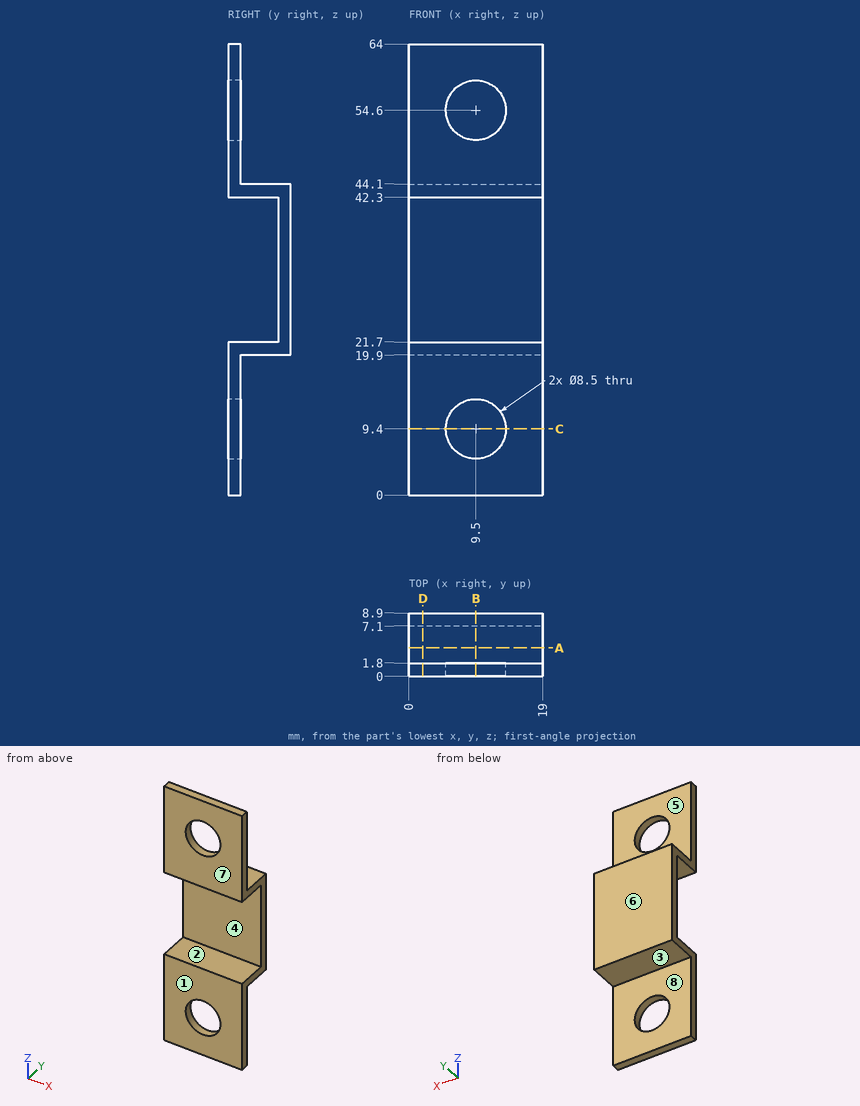
Input: dimensioned drawing with shaded views. Units: mm. Origin: part minimum x, y, z. A direction names the side the tool comes from. Give positions to 0.01 mm unless a question says otherwise; leave off trailing zeros. Loops run counter-clockwise (first coordinate to the right, second up) from the corner with the lowest first, then second, coordinate; pieces in that order, holes last. Notation, with made-up numbers: (-8.5, 42.25) -> (23.5, 42.25) arc R14 ccw to (23.5, 47.25) -> close; hole circle Ø8 at (29, 44.5). An arc over 180 degrees is marked (long way). Use a Markdown table: item, result. Add a question column.
1) Section query D-D, the plane x = 2. Return the cut outline in (y, z).
2) Section query C-C, the plane z = 9.4. Return the cut outline in (x, y), then the cut area to 3 significant figures.
3) Line query: line 1 along Z through (x, y) = (10.5, 1); line 2 along Z through (x, y) = (9.25, 4.5); line 3 along X through (y, z) = (1.45, 9.4). Output: solid intervals per line, ascending. Write a range as [from, to].
4) Section query A-A, the plane y = 4. Return the cut outline in (x, z), then the cut area to 3 significant figures.
5) Reachability of the marked faces 4, 5, 6, 7 and 8 from +Z, -Z, +X, -X, +Y, -Y: full face, straight path, thin tool, end or side. Return the list, or none.
6) First-contact query: pin 1 (5.5 mm diameter, centred on x = 9, z = 9, fed in from +Y); pin 2 (1 mm diameter, centred on x = 15, y = 6.5, fed in from -Z); pin 3 (9.5 mm diameter, centred on x = 13.5, z = 30, fed in from -Y); pin 4 (1.5 mm diameter, centred on x = 6.5, z = 6.5, fed in from +Y). Flat tips, straight axial feed; report the tip coordinate or a pass-through.
7) Section query B-B, the plane x = 9.5. Return the cut outline in (y, z).
8) Pull-direction query (Z, two-part tool) for the marked faces 1, 2 and 3; classes: +Z half, -Z half, draft (parallel to the pull), parting line (faces both ways), or undercut.
Numbers:
| question | item | result |
|---|---|---|
| 1 | outline | (0, 0) -> (1.8, 0) -> (1.8, 19.9) -> (8.9, 19.9) -> (8.9, 44.1) -> (1.8, 44.1) -> (1.8, 64) -> (0, 64) -> (0, 42.3) -> (7.1, 42.3) -> (7.1, 21.7) -> (0, 21.7) -> close |
| 2 | outline | (0, 0) -> (5.25, 0) -> (5.25, 1.8) -> (0, 1.8) -> close; (13.75, 0) -> (19, 0) -> (19, 1.8) -> (13.75, 1.8) -> close |
| 2 | area | 18.9 mm2 |
| 3 | line 1 | z = [0, 5.27], [13.53, 21.7], [42.3, 50.47], [58.73, 64] |
| 3 | line 2 | z = [19.9, 21.7], [42.3, 44.1] |
| 3 | line 3 | x = [0, 5.25], [13.75, 19] |
| 4 | outline | (0, 19.9) -> (19, 19.9) -> (19, 21.7) -> (0, 21.7) -> close; (0, 42.3) -> (19, 42.3) -> (19, 44.1) -> (0, 44.1) -> close |
| 4 | area | 68.4 mm2 |
| 5 | face 4 | +X, -X, -Y |
| 5 | face 5 | +Z, +X, -X, +Y |
| 5 | face 6 | +Z, -Z, +X, -X, +Y |
| 5 | face 7 | +Z, -Z, +X, -X, -Y |
| 5 | face 8 | -Z, +X, -X, +Y |
| 6 | pin 1 | passes through |
| 6 | pin 2 | stops at z = 19.9 |
| 6 | pin 3 | stops at y = 7.1 |
| 6 | pin 4 | stops at y = 1.8 |
| 7 | outline | (0, 0) -> (1.8, 0) -> (1.8, 5.15) -> (0, 5.15) -> close; (0, 13.65) -> (1.8, 13.65) -> (1.8, 19.9) -> (8.9, 19.9) -> (8.9, 44.1) -> (1.8, 44.1) -> (1.8, 50.35) -> (0, 50.35) -> (0, 42.3) -> (7.1, 42.3) -> (7.1, 21.7) -> (0, 21.7) -> close; (0, 58.85) -> (1.8, 58.85) -> (1.8, 64) -> (0, 64) -> close |
| 8 | face 1 | draft |
| 8 | face 2 | undercut |
| 8 | face 3 | -Z half |
